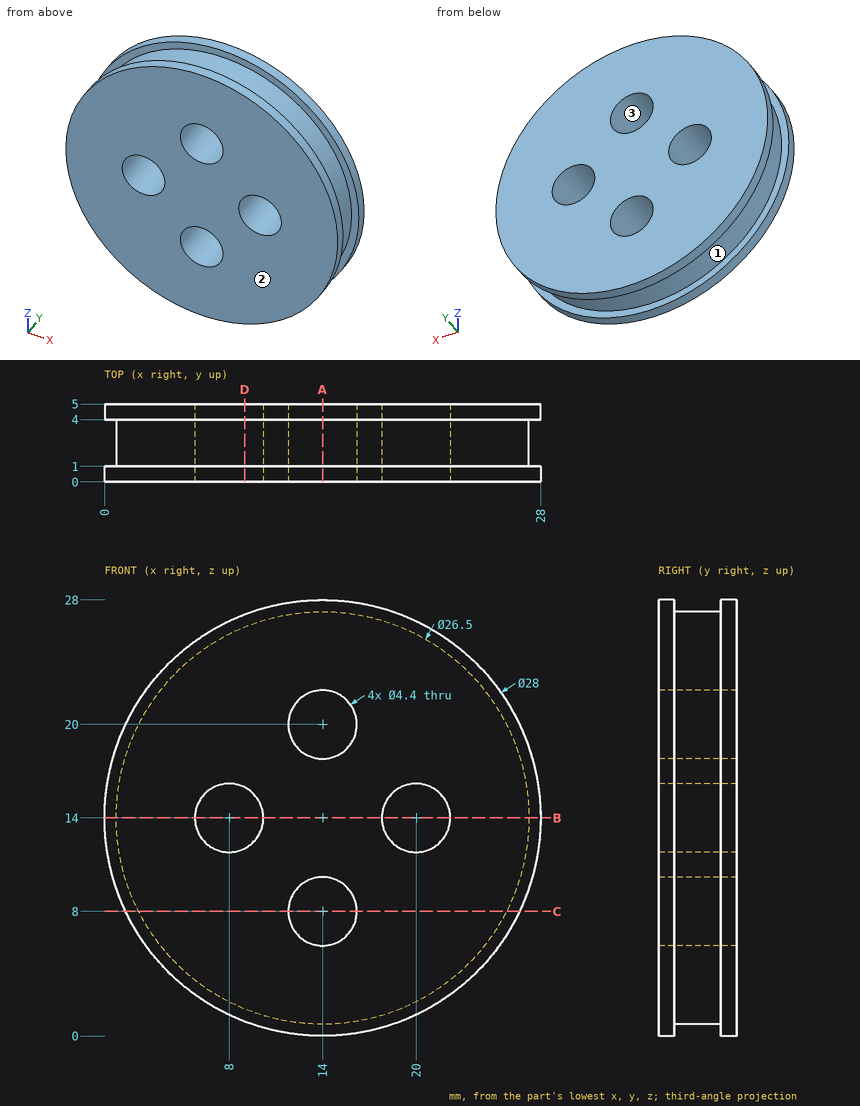
Geometry check sheet. Reference: drawing and pictorial views, mm from the part's lowest x, y, z. Round coordinates to 2 decimals unless told otherwise and drop trailing zeros. Order: outer loops, then holes, each group sorted by start corner. A loop starts at its lowest first (then second) coordinate and runs counter-clockwise, first axis right, second up. Notation, with made-up numbers: M 63,41 L 119,41 A20 ccw 119,78 Z; hole C -10.75,46.25 d10. An arc over 180 degrees is marked long. Answer in a Markdown table with one row per item.
(1) Sectioned sample at D-D, the plane x = 9. Record the cut outline in (y, z).
Responses:
| item | result |
|---|---|
| outline | M 0,0.92 L 1,0.92 L 1,1.73 L 4,1.73 L 4,0.92 L 5,0.92 L 5,12.04 L 0,12.04 Z; M 0,15.96 L 5,15.96 L 5,27.08 L 4,27.08 L 4,26.27 L 1,26.27 L 1,27.08 L 0,27.08 Z |
(2) Draft check along X on the marked faces 1, 2 and 3. Enter one of: released by +X, released by -X, zero draft, split by the parting line, or undercut.
Responses:
| item | result |
|---|---|
| face 1 | split by the parting line |
| face 2 | zero draft |
| face 3 | undercut |
(3) Sectioned sample at B-B, the plane z = 14. Record the cut outline in (x, y).
Responses:
| item | result |
|---|---|
| outline | M 0,0 L 5.8,0 L 5.8,5 L 0,5 L 0,4 L 0.75,4 L 0.75,1 L 0,1 Z; M 10.2,0 L 17.8,0 L 17.8,5 L 10.2,5 Z; M 22.2,0 L 28,0 L 28,1 L 27.25,1 L 27.25,4 L 28,4 L 28,5 L 22.2,5 Z |
(4) Go/stop test with flat-tipped pins: P1, Ø1.5, axis at y = 2.5, z = 19.5, coming from the -X side; P2, Ø3.5, axis at x = 14, z = 8, coming from the +Y side; P3, Ø1.5, axis at y = 1.5, z = 3, coming from the -X side; P4, Ø2, axis at y = 2.5, z = 13.5, coming from the -X side. Record where each tip stops, or that it passes through.
Responses:
| item | result |
|---|---|
| P1 | stops at x = 1.63 |
| P2 | passes through |
| P3 | stops at x = 4.67 |
| P4 | stops at x = 0.75 |
(5) Scan lines: probe 1 along X at (y, z) = (2.3, 14); probe 2 along Z at (x, y) = (12, 3.3). Record each from-to range of solid material in increasing order. Write a range as from..to.
Responses:
| item | result |
|---|---|
| probe 1 | x = 0.75..5.8, 10.2..17.8, 22.2..27.25 |
| probe 2 | z = 0.9..7.08, 8.92..19.08, 20.92..27.1 |
(6) Sectioned sample at C-C, the plane z = 8. Record the cut outline in (x, y).
Responses:
| item | result |
|---|---|
| outline | M 1.35,0 L 11.8,0 L 11.8,5 L 1.35,5 L 1.35,4 L 2.19,4 L 2.19,1 L 1.35,1 Z; M 16.2,0 L 26.65,0 L 26.65,1 L 25.81,1 L 25.81,4 L 26.65,4 L 26.65,5 L 16.2,5 Z |
(7) Sectioned sample at A-A, the plane x = 14. Record the cut outline in (y, z), and give its area (3 significant figures).
Responses:
| item | result |
|---|---|
| outline | M 0,0 L 1,0 L 1,0.75 L 4,0.75 L 4,0 L 5,0 L 5,5.8 L 0,5.8 Z; M 0,10.2 L 5,10.2 L 5,17.8 L 0,17.8 Z; M 0,22.2 L 5,22.2 L 5,28 L 4,28 L 4,27.25 L 1,27.25 L 1,28 L 0,28 Z |
| area | 91.5 mm² |
